For this review, take the finished solid that the model builds, in its own axes (mm). A direction names the side the tool comes from. Coordinates: 2 decimals unless noted, no trailing zeros. Order: outer loops, then holes, each group sorted by start corner. A loop starts at its lowest first (then second) coordinate and runs counter-clockwise, first axis right, second up. Notation, with made-up numbers: (2.5, -39.75) -> (37.5, -39.75) arc R31 cw to (37.5, -1.75) -> close; hole circle Ø3 at (-13.75, 50.25). An arc over 180 degrees is marked (long way). Return JSON: item names as keys, results as strings. Group by question number.
Item 1: Insertion check: pin 1 (12 mm diameter, centred on x = 19, y = 23.5, fed in from +Z); pin 2 (8 mm diameter, centred on x = 7, y = 24, fed in from +Z); pin 3 (8 mm diameter, centred on y = 7, z = 13.5, fed in from -X); pin 4 (6 mm diameter, centred on y = 12.5, z = 54, fed in from +X). Each pin has a flat end and moves straight along its axis. Give the tip position at first contact, or say it passes through.
Item 2: Draft analysis for pull direction Y (two halves, no side actions). For faces 1 (the flat face through (19.799, 9.835, 32.115)), 2 (the cylindrical face through (22.56, 5.65, 2.46)), 3 (the flat face through (8.969, 20.203, 32.115)), state which applies: +Y half, -Y half, draft (parallel to the pull), parting line (faces both ways), or undercut.
Item 3: Take a section at C-C (x = 14). Write out the cut boundary in (y, z), then the cut area to 3 significant figures.
Item 4: Machinability: for faces 4 (the flat face through (23, 5, 5)), 5 (the cylindrical face through (15.82, 11.78, 50.14)), 6 (the flat face through (4, 23, 5)), 7 (the flat face through (14, 15, 60)), which of the approach directions +Z, -Z, +X, -X, +Y, -Y give a long, thin tool a straight path to every point of the face, cutting with its end or side? Answer none if there is none.
Item 5: Take a section at B-B (z = 50.5). Write out the cut boundary in (x, y), then the cut area to 3 significant figures.
Item 6: Take a section at D-D (z = 32.5). Write out the cut boundary in (x, y).
Item 7: For line 1 along Z through (x, y) = (3.25, 24.25); line 2 along Z through (x, y) = (12, 18.5); line 3 along X through (y, z) = (17.5, 54), list the stretches that pass through material, from the lowest coordinate up.
Item 8: Take a section at A-A (y = 18.25). Write out the cut boundary in (x, z), then the cut area to 3 significant figures.
Autodesk Inventor part; units mm, degrees
ref_plane "YZ Plane" through (0, 0, 0) normal (1, 0, 0) x (0, 1, 0)
ref_plane "XZ Plane" through (0, 0, 0) normal (0, 1, 0) x (-1, 0, 0)
ref_plane "XY Plane" through (0, 0, 0) normal (0, 0, 1) x (1, 0, 0)
ref_plane "Arbeitsebene1" through (0, 0, 0) normal (0, 0, 1) x (1, 0, 0)
sketch "Skizze1" plane through (0, 0, 0) normal (0, 0, 1) x (1, 0, 0)
  circle A0 centre (-8.37, 7.9978) radius 1.4
  circle A1 centre (8.3745, -8.0022) radius 1.4
  spline S0 degree 2 poles (24.1427, 2.2394) (24.731, 1.8489) (25.3785, 0.5587) (25.3785, -0.3311) knots 0 0 0 1 2 2 2
  spline S1 degree 2 poles (25.3785, -0.3311) (25.3785, -1.1665) (24.7013, -2.5111) (24.1328, -2.8868) knots 0 0 0 1 2 2 2
  spline S2 degree 2 poles (24.1328, -2.8868) (23.6682, -3.1784) (22.7141, -3.3761) (21.9726, -3.3761) knots 0 0 0 1 2 2 2
  line L0 (21.9726, -3.3761) -> (20.5687, -3.3761)
  line L1 (20.5687, -3.3761) -> (20.5687, 2.7239)
  line L2 (20.5687, 2.7239) -> (21.9578, 2.7239)
  spline S3 degree 2 poles (21.9578, 2.7239) (22.8179, 2.7239) (23.7967, 2.4668) (24.1427, 2.2394) knots 0 0 0 1 2 2 2
  spline S4 degree 2 poles (19.1896, -2.9312) (18.8979, -3.1982) (18.1564, -3.4849) (17.5978, -3.4849) knots 0 0 0 1 2 2 2
  spline S5 degree 2 poles (17.5978, -3.4849) (16.9354, -3.4849) (16.0061, -3.2081) (15.5958, -3.0103) knots 0 0 0 1 2 2 2
  line L3 (15.5958, -3.0103) -> (15.5958, -1.992)
  line L4 (15.5958, -1.992) -> (15.6551, -1.992)
  spline S6 degree 2 poles (15.6551, -1.992) (16.0555, -2.3677) (17.0689, -2.783) (17.5385, -2.783) knots 0 0 0 1 2 2 2
  spline S7 degree 2 poles (17.5385, -2.783) (18.2108, -2.783) (18.8979, -2.2244) (18.8979, -1.7646) knots 0 0 0 1 2 2 2
  spline S8 degree 2 poles (18.8979, -1.7646) (18.8979, -1.3988) (18.5371, -0.9441) (18.1465, -0.8304) knots 0 0 0 1 2 2 2
  spline S9 degree 2 poles (18.1465, -0.8304) (17.8648, -0.7513) (17.3952, -0.6425) (17.0442, -0.5535) knots 0 0 0 1 2 2 2
  spline S10 degree 2 poles (17.0442, -0.5535) (16.7278, -0.4695) (16.2285, -0.2174) (16.0358, -0.0147) knots 0 0 0 1 2 2 2
  spline S11 degree 2 poles (16.0358, -0.0147) (15.8479, 0.188) (15.6403, 0.7317) (15.6403, 1.0876) knots 0 0 0 1 2 2 2
  spline S12 degree 2 poles (15.6403, 1.0876) (15.6403, 1.8291) (16.797, 2.8326) (17.6918, 2.8326) knots 0 0 0 1 2 2 2
  spline S13 degree 2 poles (17.6918, 2.8326) (18.2059, 2.8326) (19.1154, 2.6299) (19.5059, 2.4371) knots 0 0 0 1 2 2 2
  line L5 (19.5059, 2.4371) -> (19.5059, 1.4683)
  line L6 (19.5059, 1.4683) -> (19.4466, 1.4683)
  spline S14 degree 2 poles (19.4466, 1.4683) (19.155, 1.7352) (18.2454, 2.1307) (17.7461, 2.1307) knots 0 0 0 1 2 2 2
  spline S15 degree 2 poles (17.7461, 2.1307) (17.1826, 2.1307) (16.4856, 1.6017) (16.4856, 1.1717) knots 0 0 0 1 2 2 2
  spline S16 degree 2 poles (16.4856, 1.1717) (16.4856, 0.7861) (16.8959, 0.3264) (17.2815, 0.2226) knots 0 0 0 1 2 2 2
  spline S17 degree 2 poles (17.2815, 0.2226) (17.5385, 0.1534) (18.285, -0.0246) (18.5321, -0.0988) knots 0 0 0 1 2 2 2
  spline S18 degree 2 poles (18.5321, -0.0988) (19.1599, -0.2915) (19.7432, -1.0676) (19.7432, -1.6361) knots 0 0 0 1 2 2 2
  spline S19 degree 2 poles (19.7432, -1.6361) (19.7432, -1.997) (19.4516, -2.689) (19.1896, -2.9312) knots 0 0 0 1 2 2 2
  line L7 (-17.7002, -6.4434) -> (-23.8502, -6.4434)
  arc A2 (-23.8502, -6.4434) -> (-24.8892, -7.3274) centre (-23.8502, -7.496) ccw
  arc A3 (-25.1732, 6.2825) -> (-24.1417, 5.4391) centre (-24.1417, 6.4917) ccw
  line L8 (-24.1417, 5.4391) -> (-17.7002, 5.4391)
  arc A4 (-15.7528, 3.4917) -> (-17.7002, 5.4391) centre (-17.7002, 3.4917) ccw
  line L9 (-15.7528, 3.4917) -> (-15.7528, -4.496)
  arc A5 (-17.7002, -6.4434) -> (-15.7528, -4.496) centre (-17.7002, -4.496) ccw
  circle A6 centre (-16.3217, -17.1216) radius 2.05
  circle A7 centre (6.1284, 23.0203) radius 2.05
  circle A8 centre (22.752, 7.1358) radius 2.05
  circle A9 centre (-9.4998, -11.0022) radius 4
  circle A10 centre (0.0001, -0.0022) radius 7.5
  circle A11 centre (0, 0) radius 26.963
  circle A12 centre (0, 0) radius 20.963
  line L10 (1.3131, 26.931) -> (1.0209, 20.9381)
  line L11 (20.8731, 1.9397) -> (26.8473, 2.4948)
  circle A13 centre (6.1284, 23.0203) radius 1.5
  circle A14 centre (22.752, 7.1358) radius 1.5
  line L12 (1.0209, 20.9381) -> (20.8731, 1.9397)
  circle A15 centre (-13.4016, 13.4684) radius 4
  circle A16 centre (13.3298, -13.5395) radius 4
  line L13 (-25.1732, 9.0483) -> (-25.1732, 6.2825)
  line L14 (-24.8892, -7.3274) -> (-24.8892, -9.8026)
  arc A17 (-24.8892, -9.8026) -> (-25.1732, 9.0483) centre (0, 0) ccw
  point P0 (0, 0)
  point P1 (20.7853, 2.7239)
  point P2 (24.1373, 2.243)
  point P3 (20.5687, 2.2309)
  dimension "d1" = 6
  dimension "d2" = 5
  dimension "d3" = 5
  dimension "d6" = 3
  dimension "d7" = 3
extrude "Extrusion1" add sketch "Skizze1" along normal blind 5 contours L11 A12 L2 S3 | S3 L2 A12 L10 A17 L11 | L12 L1 L2 A12 | A17 L10 A11 L11 | L2 L1 L12 A12 | A7 | A8
fillet "Rundung1" radius 2 4 edges at (1.0209, 20.9381, 2.5) (1.3131, 26.931, 2.5) (20.8731, 1.9397, 2.5) (26.8473, 2.4948, 2.5)
sketch "Skizze2" plane through (0, 0, 5) normal (0, 0, 1) x (1, 0, 0)
  arc A0 (24.776, 2.3024) -> (26.5611, 4.6378) centre (24.5909, 4.2938) ccw
  arc A1 (26.5611, 4.6378) -> (3.4665, 26.7392) centre (0, 0) ccw
  arc A2 (3.4665, 26.7392) -> (1.2118, 24.8532) centre (3.2094, 24.7558) ccw
  line L0 (1.2118, 24.8532) -> (1.0653, 21.8495)
  arc A3 (1.0653, 21.8495) -> (1.6802, 20.3072) centre (3.063, 21.7521) ccw
  line L1 (1.6802, 20.3072) -> (20.2138, 2.5706)
  arc A4 (20.2138, 2.5706) -> (21.7817, 2.0241) centre (21.5966, 4.0155) ccw
  line L2 (21.7817, 2.0241) -> (24.776, 2.3024)
  circle A5 centre (6.1284, 23.0203) radius 1.5
  circle A6 centre (22.752, 7.1358) radius 1.5
  line L3 (1.6802, 20.3072) -> (20.2138, 2.5706)
  line L4 (5.5366, 16.6166) -> (12.4984, 23.8913)
  line L5 (16.3684, 6.2506) -> (23.3271, 13.5221)
  point P0 (0, 0)
  dimension "d9" = 4
  dimension "d10" = 4
extrude "Extrusion2" add sketch "Skizze2" along normal blind 55 contours L5 L1 L4 A1
sketch "Skizze3" plane through (0, 0, 60) normal (0, 0, 1) x (1, 0, 0)
  arc A0 (23.3271, 13.5221) -> (12.4984, 23.8913) centre (0, 0) ccw
  line L0 (12.4984, 23.8913) -> (5.5366, 16.6166)
  line L1 (5.5366, 16.6166) -> (16.3684, 6.2506)
  line L2 (16.3684, 6.2506) -> (23.3271, 13.5221)
  circle A1 centre (11.8835, 17.4634) radius 1.4
  circle A2 centre (16.9355, 12.6286) radius 1.4
  point P0 (0, 0)
  dimension "d13" = 2.8
  dimension "d14" = 2.8
  dimension "d15" = 4
  dimension "d16" = 4
  dimension "d17" = 5
  dimension "d18" = 5
extrude "Extrusion3" cut sketch "Skizze3" against normal blind 20 contours A1 | A2
properties part number "IM_Matchboxscope_Laserholder"
Findings below:
{
 "1": {"pin 1": "stops at z = 60", "pin 2": "stops at z = 5", "pin 3": "stops at x = 11.41", "pin 4": "stops at x = 23.33"},
 "2": {"face 1": "-Y half", "face 2": "undercut", "face 3": "+Y half"},
 "3": {"outline": "(8.52, 0) -> (23.04, 0) -> (23.04, 60) -> (8.52, 60) -> close", "area": "872 mm2"},
 "4": {"face 4": "+Z, +X, -Y", "face 5": "+Z", "face 6": "+Z, -X, +Y", "face 7": "+Z, +X, -X, +Y, -Y"},
 "5": {"outline": "(5.54, 16.62) -> (16.37, 6.25) -> (23.33, 13.52) arc R26.96 ccw to (12.5, 23.89) -> close; hole circle Ø2.8 at (11.88, 17.46); hole circle Ø2.8 at (16.94, 12.63)", "area": "149 mm2"},
 "6": {"outline": "(5.54, 16.62) -> (16.37, 6.25) -> (23.33, 13.52) arc R26.96 ccw to (12.5, 23.89) -> close"},
 "7": {"line 1": "z = 0 to 5", "line 2": "z = 0 to 40", "line 3": "x = 6.38 to 10.48, 13.28 to 20.51"},
 "8": {"outline": "(3.83, 0) -> (19.85, 0) -> (19.85, 60) -> (13.04, 60) -> (13.04, 40) -> (10.73, 40) -> (10.73, 60) -> (7.1, 60) -> (7.1, 5) -> (3.83, 5) -> close", "area": "735 mm2"}
}
